Here's how the part is built. I have some questions about the finished solid (model axes, mm). Give positions to 0.01 mm unless a question says otherwise; leave off trailing zeros. Loops run counter-clockwise (first coordinate to the right, second up) from the corner with the lowest first, then second, coordinate; pieces in that order, holes last. Notation, with made-up numbers: (19, -18) - (57, -18) arc R5 cw to (57, -13) - close; hole circle Ø11 at (23.5, 74.25). An arc over 180 degrees is marked (long way). Return JSON: item names as keys, results as strings. Group by question number.
(1) If we section it at D-D (y = 3): Please give me the cut outline in (x, z), then the cut area to 3 significant figures.
(2) I need wall thicknesses on probe 1 along Z at (x, y) = (0.75, -5.5); probe 2 along X at (y, z) = (-3, 1.4); probe 3 along X at (y, z) = (-3, 0.6). Which ranges of each line are inside material? Lowest first, please. Write a range as [from, to].
(3) If we section it at A-A (y = -2.25): Please give me the cut outline in (x, z).
(4) For P1, Ø0.8, axis at x = 8, y = -3, coming from the +Z side; P2, Ø1, axis at x = -0.5, z = 1, coming from the -Y side, each with a flat end and sliding along its axis, tell me the tip position at first contact or that it passes through.
(5) If we section it at C-C (x = -0.5): Please give me the cut outline in (y, z), then the cut area to 3 significant figures.
(6) If we section it at B-B (z = 1): Please give me the cut outline in (x, y), then the cut area to 3 significant figures.
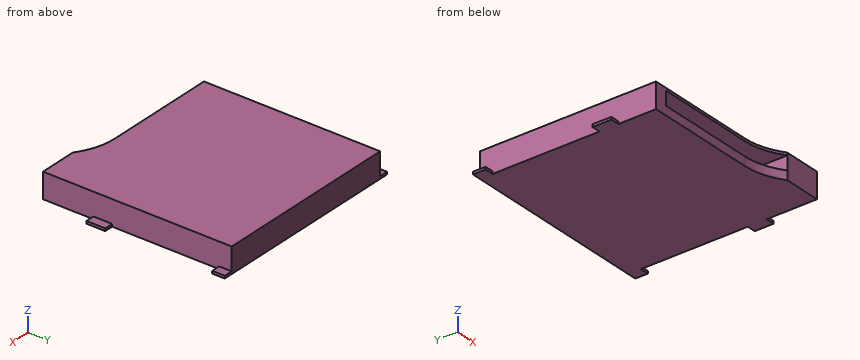
```python
from build123d import *

# Parameters (mm, degrees)
BOSS_EXTRUDE1_DEPTH = 2
SKETCH2_W           = 11
SKETCH2_H           = 1.1
CUT_EXTRUDE1_DEPTH  = 12
SKETCH3_W           = 0.7
SKETCH3_H           = 1
SKETCH3_H_2         = 1.5
BOSS_EXTRUDE2_DEPTH = 0.2


with BuildPart() as part:
    # Sketch1 → Boss-Extrude1 (new body)
    with BuildSketch(Plane.XY):
        with BuildLine():
            Line((-7.5, 7.5), (7.5, 7.5))
            Line((7.5, 7.5), (7.5, -7.5))
            Line((7.5, -7.5), (4.5, -7.5))
            add(Edge.make_bspline(
                [(1.5, -6.5), (3.08113883, -6.5), (4.5, -7.5)],
                knots=[0, 0, 0, 1, 1, 1], degree=2))
            Line((1.5, -6.5), (-7.5, -6.5))
            Line((-7.5, -6.5), (-7.5, 7.5))
        make_face()
    extrude(amount=BOSS_EXTRUDE1_DEPTH)

    # Sketch2 → Cut-Extrude1 (cut)
    with BuildSketch(Plane.XZ.offset(7.5)):
        with Locations((-1, 1.25)):
            Rectangle(SKETCH2_W, SKETCH2_H)
    extrude(amount=-CUT_EXTRUDE1_DEPTH, mode=Mode.SUBTRACT)

    # Sketch3 → Boss-Extrude2 (add)
    with BuildSketch(Plane.XY):
        with Locations((7.85, 7)):
            Rectangle(SKETCH3_W, SKETCH3_H)
        with Locations((-7.85, 7)):
            Rectangle(SKETCH3_W, SKETCH3_H)
        with Locations((-7.85, -2.75)):
            Rectangle(SKETCH3_W, SKETCH3_H_2)
        with Locations((7.85, -2.75)):
            Rectangle(SKETCH3_W, SKETCH3_H_2)
    extrude(amount=BOSS_EXTRUDE2_DEPTH)


solid = part.part
```
Values:
{
 "1": {"outline": "(-7.5, 0) - (7.5, 0) - (7.5, 2) - (-7.5, 2) - close; hole (-6.5, 0.7) - (4.5, 0.7) - (4.5, 1.8) - (-6.5, 1.8) - close", "area": "17.9 mm2"},
 "2": {"probe 1": "[0, 0.7], [1.8, 2]", "probe 2": "[-7.5, -6.5], [4.5, 7.5]", "probe 3": "[-7.5, 7.5]"},
 "3": {"outline": "(-8.2, 0) - (8.2, 0) - (8.2, 0.2) - (7.5, 0.2) - (7.5, 2) - (-7.5, 2) - (-7.5, 0.2) - (-8.2, 0.2) - close; hole (-6.5, 0.7) - (4.5, 0.7) - (4.5, 1.8) - (-6.5, 1.8) - close"},
 "4": {"P1": "z = 0.2", "P2": "y = -6.5"},
 "5": {"outline": "(-6.5, 0) - (7.5, 0) - (7.5, 2) - (-6.5, 2) - (-6.5, 1.8) - (4.5, 1.8) - (4.5, 0.7) - (-6.5, 0.7) - close", "area": "15.9 mm2"},
 "6": {"outline": "(-7.5, -6.5) - (-6.5, -6.5) - (-6.5, 4.5) - (4.5, 4.5) - (4.5, -7.5) - (7.5, -7.5) - (7.5, 7.5) - (-7.5, 7.5) - close", "area": "92.0 mm2"}
}
